Could you check a few things on this drawing? It's one solid part, dimensions in mm from its lowest x, y, z. A direction names the side the tool comes from. Round coordinates to 2 decimals unless told otherwise and drop trailing zeros. Write each loop counter-clockwise with the first axis right and the second up, starting at its lowest first coordinate (ties: lowest second). Pieces come first, ordered by that corner, then holes. Notation, with made-up numbers: (69.5, 39) -> (93.5, 39) arc R25 cw to (93.5, 68) -> close; hole circle Ø2 at (7, -36). An arc over 180 degrees is marked (long way). Return JSON: item names as keys, results as strings.
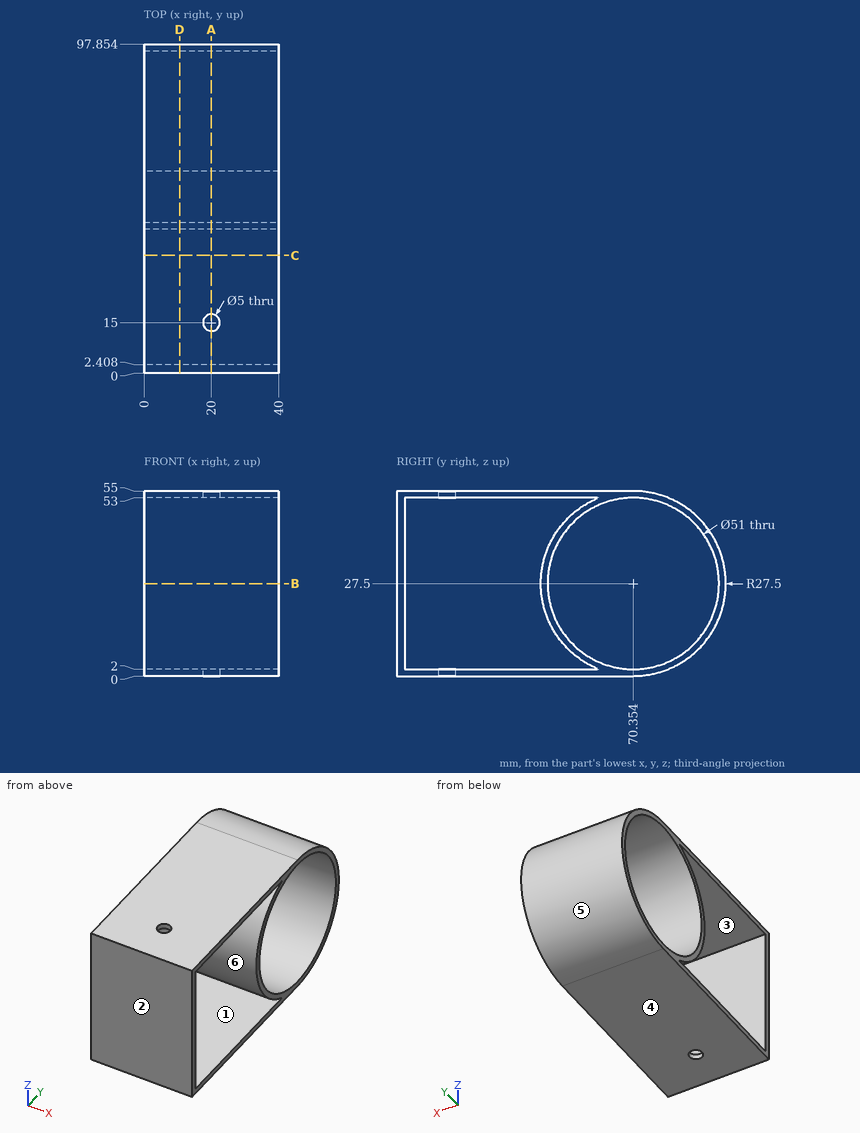
1) For the marked faces 1 and 2, which set-ups out of +Z, -Z, +X, -X, +Y, -Y let a thin tool reach every point of the face, with its end or its side?
Return value:
{"face 1": "+X, -X", "face 2": "+Z, -Z, +X, -X, -Y"}
2) Will these pins go through, and if not, where does the flat tip stop? pin 1 Ø20 at (x, z) = (22, 16.5) entering from +Y; pin 2 Ø5 at (x, y) = (35.5, 79) entering from -Z (1 decimal); pin 3 Ø3 at (x, y) = (20, 15) entering from -Z; pin 4 Ø5 at (x, z) = (7.5, 48) entering from +Y (1 decimal).
Return value:
{"pin 1": "y = 97.84", "pin 2": "z = 0.7", "pin 3": "through", "pin 4": "y = 91.1"}
3) I want a section at A-A, the plane x = 20. Please give me the cut outline in (y, z) (1 decimal).
Return value:
{"outline": "(0, 0) -> (12.5, 0) -> (12.5, 2) -> (2.4, 2) -> (2.4, 53) -> (12.5, 53) -> (12.5, 55) -> (0, 55) -> close; (17.5, 0) -> (70.4, 0) arc R27.5 ccw to (70.4, 55) -> (17.5, 55) -> (17.5, 53) -> (60.1, 53) arc R27.5 ccw to (60.1, 2) -> (17.5, 2) -> close; hole circle Ø51 at (70.4, 27.5)"}
4) If I drill on probe 1 along Z at (x, y) = (30, 55.5) (1 decimal); probe 2 along Y at (x, z) = (29, 40); probe 3 along Z at (x, y) = (13, 25.5), over which ranges is the centre line in solid material (lowest first)? Write a range as [from, to].
Return value:
{"probe 1": "[0, 2], [4.4, 6.8], [48.2, 50.6], [53, 55]", "probe 2": "[0, 2.41], [45.86, 48.13], [92.58, 94.85]", "probe 3": "[0, 2], [53, 55]"}
5) Thinking about a two-plate mould opening in Z: for the marked faces 3, 4, 5 and 6, which applies, pulls with the +Z half, pulls with the -Z half, needs draft (parallel to the pull), parting line crosses it, or undercut?
Return value:
{"face 3": "undercut", "face 4": "pulls with the -Z half", "face 5": "parting line crosses it", "face 6": "undercut"}
6) I want a section at C-C, the plane y = 35. Please give me the cut outline in (x, z).
Return value:
{"outline": "(0, 0) -> (40, 0) -> (40, 2) -> (0, 2) -> close; (0, 53) -> (40, 53) -> (40, 55) -> (0, 55) -> close"}
7) I want a section at B-B, the plane z = 27.5. Please give me the cut outline in (x, y) (1 decimal).
Return value:
{"outline": "(0, 0) -> (40, 0) -> (40, 2.4) -> (0, 2.4) -> close; (0, 42.9) -> (40, 42.9) -> (40, 44.9) -> (0, 44.9) -> close; (0, 95.9) -> (40, 95.9) -> (40, 97.9) -> (0, 97.9) -> close"}
8) I want a section at D-D, the plane x = 10.5. Please give me the cut outline in (y, z) (1 decimal).
Return value:
{"outline": "(0, 0) -> (70.4, 0) arc R27.5 ccw to (70.4, 55) -> (0, 55) -> close; hole (2.4, 2) -> (60.1, 2) arc R27.5 cw to (60.1, 53) -> (2.4, 53) -> close; hole circle Ø51 at (70.4, 27.5)"}
